Input: part model. Units: mm. Frame: model coordinates. A direction names the side the tool comes from. Give positions to 0.01 mm unless a question says otherwise; leave off trailing zeros. Write each loop counter-clockwise with the first axis right and the second up, starting at its lowest first coordinate (ties: lowest second). Pieces come first, ordered by that corner, then holes.
```python
from build123d import *
from build123d.topology import SkipClean

# Parameters (mm, degrees)
SKETCH1_R           = 38.1
BOSS_EXTRUDE1_DEPTH = 12.7
SKETCH2_R           = 11.43
BOSS_EXTRUDE2_DEPTH = 73.914
FILLET1_R           = 1.27
FILLET2_R           = 1.27
FILLET3_R           = 3.81
CUT_EXTRUDE2_DEPTH  = 3.81
CUT_EXTRUDE3_DEPTH  = 3.81


with BuildPart() as part:
    # Sketch1 → Boss-Extrude1 (new body)
    with BuildSketch(Plane(origin=(0, 0, 0), x_dir=(1, 0, 0), z_dir=(0, 1, 0))):
        with Locations(Location((0, 0, 0), (0, 0, 270))):
            Circle(SKETCH1_R)
    extrude(amount=BOSS_EXTRUDE1_DEPTH)

    # Sketch2 → Boss-Extrude2 (add)
    with BuildSketch(Plane(origin=(0, 12.7, 0), x_dir=(1, 0, 0), z_dir=(0, 1, 0))):
        with Locations(Location((0, 0, 0), (0, 0, 270))):
            Circle(SKETCH2_R)
    extrude(amount=BOSS_EXTRUDE2_DEPTH)

    # Fillet1
    fillet1_edges = [part.edges().sort_by_distance(p)[0] for p in [
        (0, 12.7, -38.1),
    ]]
    fillet(fillet1_edges, radius=FILLET1_R)

    # Fillet2
    fillet2_edges = [part.edges().sort_by_distance(p)[0] for p in [
        (0, 0, -38.1),
    ]]
    fillet(fillet2_edges, radius=FILLET2_R)

    # Fillet3
    fillet3_edges = [part.edges().sort_by_distance(p)[0] for p in [
        (0, 86.614, -11.43),
    ]]
    fillet(fillet3_edges, radius=FILLET3_R)

    # Sketch4 → Cut-Extrude2 (cut)
    with BuildSketch(Plane(origin=(0, 12.7, 0), x_dir=(-1, 0, 0), z_dir=(0, -1, 0))):
        with BuildLine():
            ThreePointArc((-12.106701586, -25.883554657), (-18.053418689, -24.924958375), (-13.874033018, -29.26259443))
            ThreePointArc((-13.874033018, -29.26259443), (-11.127331545, -30.41333125), (-8.286537239, -31.306892621))
            ThreePointArc((-8.286537239, -31.306892621), (-5.957511953, -29.952754069), (-7.311650505, -27.623728783))
            ThreePointArc((-7.311650505, -27.623728783), (-9.748084477, -26.860853933), (-12.106701586, -25.883554657))
        make_face()
        with BuildLine():
            ThreePointArc((28.469166667, 2.457066199), (30.612356486, -3.172240023), (32.279166667, 2.616032168))
            ThreePointArc((32.279166667, 2.616032168), (31.902383248, 5.570113831), (31.255832943, 8.477094553))
            ThreePointArc((31.255832943, 8.477094553), (28.918601914, 9.81702034), (27.578676126, 7.479789311))
            ThreePointArc((27.578676126, 7.479789311), (28.136224112, 4.988338171), (28.469166667, 2.457066199))
        make_face()
        with BuildLine():
            ThreePointArc((-16.36246508, 23.426488458), (-12.558937796, 28.097198398), (-18.405133648, 26.646562262))
            ThreePointArc((-18.405133648, 26.646562262), (-20.775051704, 24.843217419), (-22.969295704, 22.829798069))
            ThreePointArc((-22.969295704, 22.829798069), (-22.961089961, 20.135733729), (-20.267025621, 20.143939472))
            ThreePointArc((-20.267025621, 20.143939472), (-18.388139635, 21.872515762), (-16.36246508, 23.426488458))
        make_face()
    extrude(amount=CUT_EXTRUDE2_DEPTH, mode=Mode.SUBTRACT)

    # Sketch5 → Cut-Extrude3 (cut)
    with SkipClean():  # the faces are left unmerged after this step: merging them gives an invalid solid
        with BuildSketch(Plane(origin=(0, 8.89, 0), x_dir=(1, 0, 0), z_dir=(0, 1, 0))):
            with BuildLine():
                ThreePointArc((16.8275, -29.146084964), (17.989630657, -24.808954307), (13.6525, -23.64682365))
                ThreePointArc((13.6525, -23.64682365), (10.410740895, -25.242414683), (6.98668826, -26.396007504))
                ThreePointArc((6.98668826, -26.396007504), (4.729790674, -30.277716314), (8.611499483, -32.5346139))
                ThreePointArc((8.611499483, -32.5346139), (12.831843428, -31.112743679), (16.8275, -29.146084964))
            make_face()
            with BuildLine():
                ThreePointArc((-32.481551882, 8.809529633), (-33.360348122, 4.443669453), (-33.655, 0))
                ThreePointArc((-33.655, 0), (-30.48, -3.175), (-27.305, 0))
                ThreePointArc((-27.305, 0), (-27.065942816, 3.605241255), (-26.352957187, 7.147354231))
                ThreePointArc((-26.352957187, 7.147354231), (-28.586166833, 11.042739279), (-32.481551882, 8.809529633))
            make_face()
            with BuildLine():
                ThreePointArc((23.870052398, 23.725084267), (20.528504693, 26.669074226), (16.8275, 29.146084964))
                ThreePointArc((16.8275, 29.146084964), (12.490369343, 27.983954307), (13.6525, 23.64682365))
                ThreePointArc((13.6525, 23.64682365), (16.655201921, 21.637173428), (19.366268927, 19.248653274))
                ThreePointArc((19.366268927, 19.248653274), (23.85637616, 19.234977035), (23.870052398, 23.725084267))
            make_face()
        extrude(amount=-CUT_EXTRUDE3_DEPTH, mode=Mode.SUBTRACT)


solid = part.part
```
Q1. Pin query (flat end, axial travel): pin 1 (2 mm diameter, centred on x = -28, z = -6, fed in from -Y); pin 2 (5.5 mm diameter, centred on x = 20, z = -22.5, fed in from +Y); pin 3 (5 mm diameter, centred on x = 15.24, z = 26.4, fed in from +Y); pin 4 (10 mm diameter, centred on y = 31, z = 0.5, fed in from -X). Return the tip coordinate at first contact, or that it passes through.
Q2. Section A-A, the plane x = 0. Return the cut outline in (y, z).
Q3. Access query for faces 5 (the cylindrical face through (-33.35, 7.01, -4.51)), 6 (the cylindrical face through (9.714, 10.822, 26.873)), 7 (the flat face through (1, 0, -1)). Directions: +Z, -Z, +X, -X, +Y, -Y. A direction counts if a zero-diameter tool reaches every point of the face in a straight line with its end or side. Return the directions, or none.
Q4. Mould query, pull axis Z, two halves, no side actions, for faces 1 (the flat face through (-30, 5.08, -4)), 2 (the cylindrical face through (-23.183, 6.279, -30.235)), 3 (the cylindrical face through (10.46, 7.01, 25.22)), 4 (the flat face through (0, 86.614, 0)). Classes: +Z half, -Z half, draft (parallel to the pull), parting line (faces both ways), or undercut.
Q5. Material intervals for line 1 along Z through (x, y) = (15.24, 9.8); line 2 along X through (y, z) = (10.5, 0) (3 decimals); line 3 along Z through (x, y) = (15, 11), sorted ascending.
Q6. Section B-B, the plane y = 26. Return the cut outline in (x, z), then the cut area to 3 significant figures.
Solutions:
1. pin 1: stops at y = 0
1. pin 2: stops at y = 12.7
1. pin 3: stops at y = 5.08
1. pin 4: stops at x = -11.43
2. outline: (0, -36.83) arc R1.27 ccw to (1.27, -38.1) - (11.43, -38.1) arc R1.27 ccw to (12.7, -36.83) - (12.7, -11.43) - (82.8, -11.43) arc R3.81 ccw to (86.61, -7.62) - (86.61, 7.62) arc R3.81 ccw to (82.8, 11.43) - (12.7, 11.43) - (12.7, 36.83) arc R1.27 ccw to (11.43, 38.1) - (1.27, 38.1) arc R1.27 ccw to (0, 36.83) - close
3. face 5: none
3. face 6: +Y
3. face 7: +Z, -Z, +X, -X, -Y
4. face 1: undercut
4. face 2: parting line
4. face 3: undercut
4. face 4: draft
5. line 1: z = -34.92 to -29.57, -23.22 to 23.22, 29.57 to 34.92
5. line 2: x = -38.1 to -33.655, -27.305 to 38.1
5. line 3: z = -35.02 to -29.56, -23.23 to 23.23, 29.56 to 35.02
6. outline: circle Ø22.86 at (0, 0)
6. area: 410 mm2
